Drawing for the job (mm, zero at the part's lowest x, y, z). Coordinates: 2 decimals unless noted, no trailing zeros. Loops run counter-clockwise (first coordinate to the right, second up) from the corner with the lowest first, then second, coordinate; pieces in that order, holes last. Notation, with made-up numbers: (11, 85) - (35, 85) arc R23 cw to (35, 123) - close; hole circle Ø2 at (59.25, 75). An arc over 180 degrees is marked (long way). One line per item, written item: value.
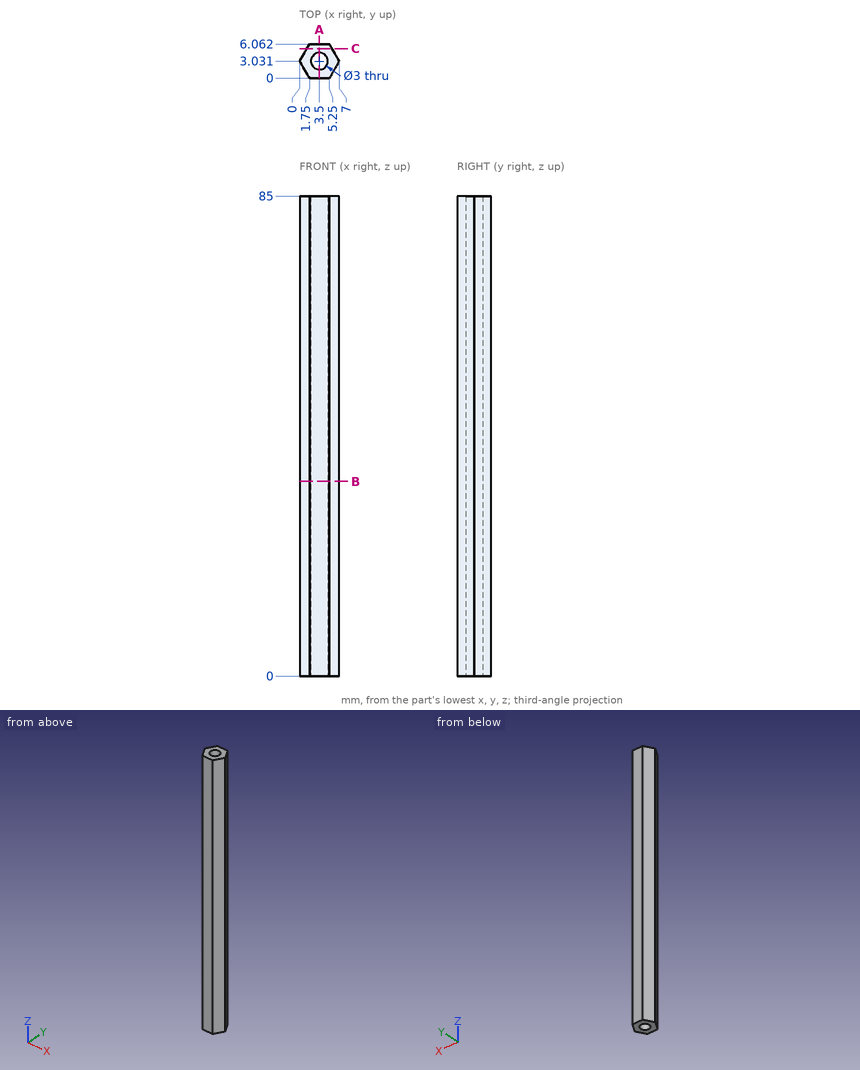
Item 1: Probe probe 1 along Y at (x, z) = (3.5, 43); probe 2 along X at (y, z) = (3, 9); probe 3 along X at (y, z) = (1.75, 17). List the from-to ranges inside material, lowest first. Write a range as from..to.
Check result:
probe 1: y = 0..1.53, 4.53..6.06
probe 2: x = 0.02..2, 5..6.98
probe 3: x = 0.74..2.72, 4.28..6.26
Item 2: Cut at C-C, the plane y = 5.25. Write the cut outline in (x, z).
Check result:
outline: (1.28, 0) - (5.72, 0) - (5.72, 85) - (1.28, 85) - close
Item 3: Cut at A-A, the plane x = 3.5. Write the cut outline in (y, z), then the cut area to 3 significant figures.
Check result:
outline: (0, 0) - (1.53, 0) - (1.53, 85) - (0, 85) - close; (4.53, 0) - (6.06, 0) - (6.06, 85) - (4.53, 85) - close
area: 260 mm^2
Item 4: Drop flat-ended pins along their axis: P1, Ø2.5, axis at x = 3.5, y = 3.03, coming from the +Z side; P2, Ø2, axis at y = 3.5, z = 71.5, coming from the -X side. Give the stop position or say it passes through.
Check result:
P1: passes through
P2: stops at x = 0
Item 5: Cut at B-B, the plane z = 34.5. Write the cut outline in (x, y).
Check result:
outline: (0, 3.03) - (1.75, 0) - (5.25, 0) - (7, 3.03) - (5.25, 6.06) - (1.75, 6.06) - close; hole circle Ø3 at (3.5, 3.03)
